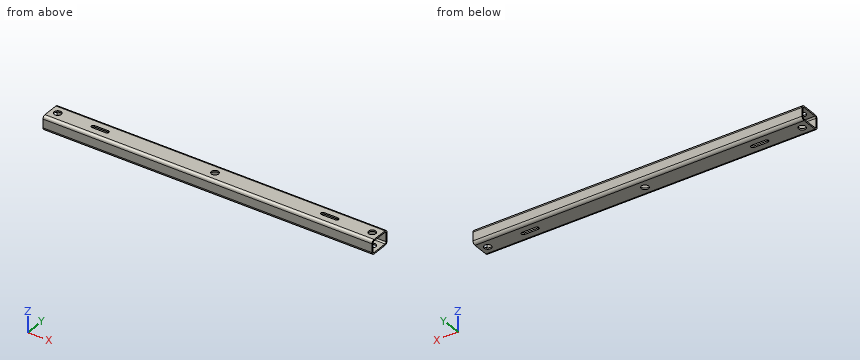
```python
from build123d import *

# Parameters (mm, degrees)
SKETCH1_W               = 2300
SKETCH1_H               = 150
BOSS_EXTRUDE1_DEPTH     = 100
CUT_EXTRUDE1_DEPTH      = 2304.394234602
CUT_EXTRUDE1_DEPTH_BACK = 2304.394234602
SKETCH3_W               = 80
SKETCH3_H               = 130
FILLET1_R               = 10
FILLET2_R               = 20
SKETCH4_R               = 25
CUT_EXTRUDE2_DEPTH      = 1157.773530126
CUT_EXTRUDE3_DEPTH      = 1157.773530126


with BuildPart() as part:
    # Sketch1 → Boss-Extrude1 (new body)
    with BuildSketch(Plane.XY):
        Rectangle(SKETCH1_W, SKETCH1_H)
    extrude(amount=BOSS_EXTRUDE1_DEPTH)

    # Sketch3 → Cut-Extrude1 (cut, two sides: drawn at the far end of the back side and taken through both)
    with BuildSketch(Plane.ZY.offset(1150).offset(-CUT_EXTRUDE1_DEPTH_BACK)):
        with Locations((50, 0)):
            Rectangle(SKETCH3_W, SKETCH3_H)
    extrude(amount=CUT_EXTRUDE1_DEPTH + CUT_EXTRUDE1_DEPTH_BACK, mode=Mode.SUBTRACT)

    # Fillet1
    fillet1_edges = [part.edges().sort_by_distance(p)[0] for p in [
        (0, -65, 90),
        (0, -65, 10),
        (0, 65, 10),
        (0, 65, 90),
    ]]
    fillet(fillet1_edges, radius=FILLET1_R)

    # Fillet2
    fillet2_edges = [part.edges().sort_by_distance(p)[0] for p in [
        (0, 75, 100),
        (0, 75, 0),
        (0, -75, 0),
        (0, -75, 100),
    ]]
    fillet(fillet2_edges, radius=FILLET2_R)

    # Sketch4 → Cut-Extrude2 (cut, through all)
    with BuildSketch(Plane(origin=(0, 0, 0), x_dir=(-1, 0, 0), z_dir=(0, 0, -1))):
        Circle(SKETCH4_R)
        with Locations((-1098.86, 0)):
            Circle(SKETCH4_R)
        with Locations((1098.86, 0)):
            Circle(SKETCH4_R)
    extrude(amount=-CUT_EXTRUDE2_DEPTH, mode=Mode.SUBTRACT)

    # Sketch5 → Cut-Extrude3 (cut, through all)
    with BuildSketch(Plane(origin=(0, 0, 0), x_dir=(-1, 0, 0), z_dir=(0, 0, -1))):
        with BuildLine():
            Line((-851.045, 12.91), (-753.695, 12.91))
            ThreePointArc((-753.695, 12.91), (-740.785, 0), (-753.695, -12.91))
            Line((-753.695, -12.91), (-851.045, -12.91))
            ThreePointArc((-851.045, -12.91), (-863.955, 0), (-851.045, 12.91))
        make_face()
        with BuildLine():
            Line((851.045, 12.91), (753.695, 12.91))
            ThreePointArc((753.695, 12.91), (740.785, 0), (753.695, -12.91))
            Line((753.695, -12.91), (851.045, -12.91))
            ThreePointArc((851.045, -12.91), (863.955, 0), (851.045, 12.91))
        make_face()
    extrude(amount=-CUT_EXTRUDE3_DEPTH, mode=Mode.SUBTRACT)


solid = part.part
```
Input: part model. Units: mm. Frame: model coordinates. Round coordinates to 2 decimals unless told otherwise and drop trailing zeros. Loops run counter-clockwise (first coordinate to the right, second up) from the corner with the lowest first, then second, coordinate; pieces in that order, holes last. Notation, with made-up numbers: (41.25, 38) -> (93.25, 38) arc R23 ccw to (93.25, 75) -> close; hole circle Ø9 at (-14.5, 70.5). An arc over 180 degrees is marked (long way). Write each question's results on one line, items separated by ' | '.
1. Ray query, line 1 (Z direction, x = 415.5, y = 43); line 2 (Y direction, x = -826.5, z = 25); line 3 (Z direction, x = 687, y = 57). Return the intervals inside material, ascending. Write a range as from..to.
Geometry results:
line 1: 0..10, 90..100 | line 2: -75..-65, 65..75 | line 3: 0.1..10.2, 89.8..99.9
2. First-contact query: P1, Ø3, axis at x = -793, z = 97.5, coming from the +Y side; P2, Ø11, axis at x = 788.5, z = 3.5, coming from the -Y side; P3, Ø8, axis at x = -825, z = 4.5, coming from the -Y side. Flat tips, straight axial feed; report the tip coordinate or a pass-through.
Geometry results:
P1: y = 67 | P2: y = -71.7 | P3: y = -71.36
3. Section A-A (x = 291). Return loops of the section in (y, z).
Geometry results:
outline: (-75, 20) arc R20 ccw to (-55, 0) -> (55, 0) arc R20 ccw to (75, 20) -> (75, 80) arc R20 ccw to (55, 100) -> (-55, 100) arc R20 ccw to (-75, 80) -> close; hole (-65, 20) arc R10 ccw to (-55, 10) -> (55, 10) arc R10 ccw to (65, 20) -> (65, 80) arc R10 ccw to (55, 90) -> (-55, 90) arc R10 ccw to (-65, 80) -> close
4. Section B-B (z = 52.5). Return loops of the section in (x, y), and give its area (3 significant figures).
Geometry results:
outline: (-1150, -75) -> (1150, -75) -> (1150, -65) -> (-1150, -65) -> close; (-1150, 65) -> (1150, 65) -> (1150, 75) -> (-1150, 75) -> close | area: 46,000 mm2
5. Section C-C (x = -1098.86). Return loops of the section in (y, z), and give its area (3 significant figures).
Geometry results:
outline: (-75, 20) arc R20 ccw to (-55, 0) -> (-25, 0) -> (-25, 10) -> (-55, 10) arc R10 cw to (-65, 20) -> (-65, 80) arc R10 cw to (-55, 90) -> (-25, 90) -> (-25, 100) -> (-55, 100) arc R20 ccw to (-75, 80) -> close; (25, 0) -> (55, 0) arc R20 ccw to (75, 20) -> (75, 80) arc R20 ccw to (55, 100) -> (25, 100) -> (25, 90) -> (55, 90) arc R10 cw to (65, 80) -> (65, 20) arc R10 cw to (55, 10) -> (25, 10) -> close | area: 3,340 mm2
